Geometry: final body of the model. Coordinates: model frame, mm. A direction names the side the tool comes from. Give positions to 0.01 mm unless a question says otherwise; leave off trailing zeros. Order: outer loops, then holes, each group sorted by start corner. A loop starts at its lowest first (then second) coordinate and runs counter-clockwise, first axis right, second up. Notation, with made-up numbers: (35, 62) - (53, 62) arc R27 ccw to (53, 90) - close; hole circle Ø6 at (30, 77). An arc over 180 degrees is marked (long way). Use one line per item in the form item = value.
from build123d import *

# Parameters (mm, degrees)
ESBO_O1_R                = 3.9
ESBO_O1_R_2              = 1.55
RESSALTO_EXTRUS_O1_DEPTH = 6
ESBO_O2_R                = 7.5
ESBO_O2_R_2              = 1.55
RESSALTO_EXTRUS_O2_DEPTH = 1
CORTE_EXTRUS_O1_DEPTH    = 3
FILETE1_R                = 1


with BuildPart() as part:
    # Esboço1 → Ressalto-extrusão1 (new body)
    with BuildSketch(Plane(origin=(0, 0, 0), x_dir=(0, 0, -1), z_dir=(1, 0, 0))):
        Circle(ESBO_O1_R)
        Circle(ESBO_O1_R_2, mode=Mode.SUBTRACT)
    extrude(amount=RESSALTO_EXTRUS_O1_DEPTH)

    # Esboço2 → Ressalto-extrusão2 (add)
    with BuildSketch(Plane(origin=(6, 0, 0), x_dir=(0, 0, -1), z_dir=(1, 0, 0))):
        Circle(ESBO_O2_R)
        Circle(ESBO_O2_R_2, mode=Mode.SUBTRACT)
    extrude(amount=RESSALTO_EXTRUS_O2_DEPTH)

    # Esboço3 → Corte-extrusão1 (cut)
    with BuildSketch(Plane.ZY):
        Polygon((1.703183294, -2.95), (3.406366588, 0), (1.703183294, 2.95), (-1.703183294, 2.95), (-3.406366588, 0), (-1.703183294, -2.95), align=None)
    extrude(amount=-CORTE_EXTRUS_O1_DEPTH, mode=Mode.SUBTRACT)

    # Filete1
    filete1_edges = [part.edges().sort_by_distance(p)[0] for p in [
        (6, 0, 3.9),
    ]]
    fillet(filete1_edges, radius=FILETE1_R)


solid = part.part
(1) Ray query, line 1 along Y through (x, z) = (5.05, 0); line 2 along X through (y, z) = (-2, -6); line 3 along Z through (x, y) = (0.75, 1.5). Return the intervals inside material, ascending.
Computed values:
line_1 = -3.9 to -1.55, 1.55 to 3.9
line_2 = 6 to 7
line_3 = -3.6 to -2.54, 2.54 to 3.6
(2) Pull-direction query (Y, two-part tool) for faces 3 (the face through (6.493, 0.33, 7.493)), 4 (the face through (6, -5, -2)), 5 (the face through (4.972, -1.375, -0.715)); classes: released by +Y, released by -Y, zero draft, split by the parting line, or undercut.
Computed values:
face_3 = split by the parting line
face_4 = zero draft
face_5 = undercut
(3) Cut plane A-A on z = 0. Output: boundary loops of the cut face in (x, y).
Computed values:
outline = (0, -3.9) - (5, -3.9) arc R1 cw to (6, -4.9) - (6, -7.5) - (7, -7.5) - (7, -1.55) - (3, -1.55) - (3, -2.95) - (0, -2.95) - close; (0, 2.95) - (3, 2.95) - (3, 1.55) - (7, 1.55) - (7, 7.5) - (6, 7.5) - (6, 4.9) arc R1 cw to (5, 3.9) - (0, 3.9) - close
(4) Cut plane C-C on z = -5.5. Output: boundary loops of the cut face in (x, y), plus the area to 3 significant figures.
Computed values:
outline = (6, -5.1) - (7, -5.1) - (7, 5.1) - (6, 5.1) - close
area = 10.2 mm²
(5) Reachability of faces 1 (the face through (1.48, -1.45, -2.57)), 2 (the face through (7, 0, -2)) from +Z, -Z, +X, -X, +Y, -Y: full face, straight path, thin tool, end or side. Return the list, or none.
Computed values:
face_1 = -X
face_2 = +Z, -Z, +X, +Y, -Y
(6) Cut plane B-B on x = 0.75. Output: boundary loops of the cut face in (y, z).
Computed values:
outline = circle Ø7.8 at (0, 0); hole (-2.95, -1.7) - (0, -3.41) - (2.95, -1.7) - (2.95, 1.7) - (0, 3.41) - (-2.95, 1.7) - close
(7) Contact query for flat-ended pins moving along their axis: pin 1 Ø6 at (y, z) = (4, 1.5) entering from -X; pin 2 Ø1 at (x, z) = (3, -4) entering from +Y; pin 3 Ø2 at (y, z) = (-6, -4) entering from -X; pin 4 Ø1.8 at (y, z) = (-0.5, 1) entering from -X. Output: stop coordinate, or through.
Computed values:
pin_1 = 0
pin_2 = 1.72
pin_3 = 6
pin_4 = 3
